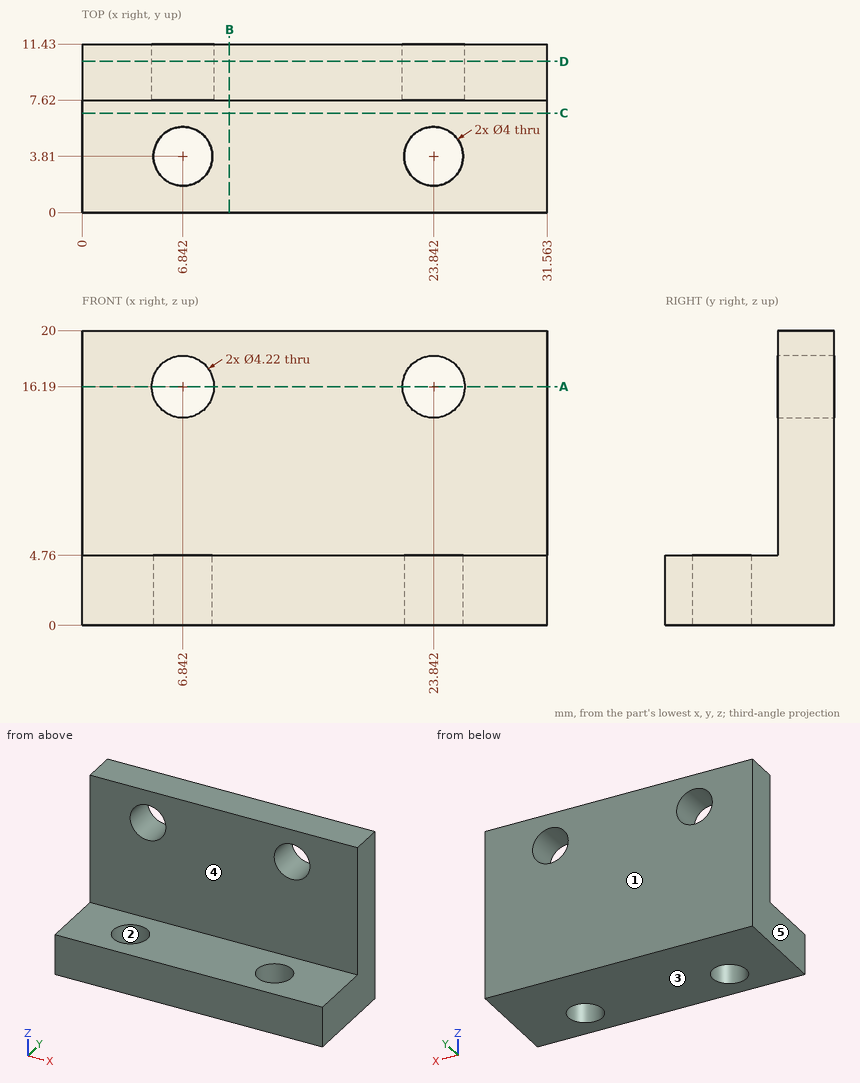
Input: dimensioned drawing with shaded views. Units: mm. Origin: part minimum x, y, z. A direction names the side the tool comes from. Round coordinates to 2 decimals unless told otherwise and drop trailing zeros. Write each loop counter-clockwise with the first axis right and the second up, starting at its lowest first coordinate (ties: lowest second). Pieces come first, ordered by that corner, then holes. Notation, with made-up numbers: (86.5, -12.5) - (136.5, -12.5) arc R18 cw to (136.5, -3.5) - close; hole circle Ø4 at (67.5, -38.5). An arc over 180 degrees is marked (long way). Write item = value, one per line.
(1) Pull-direction query (Y, two-part tool) for the marked faces 1, 2 and 3; classes: +Y half, -Y half, draft (parallel to the pull), parting line (faces both ways), or undercut.
Geometry check:
face_1 = +Y half
face_2 = undercut
face_3 = draft
(2) Contact query for a flat-ended pin moving along its axis: pin 1 Ø12 at (x, z) = (13, 11) entering from -Y. Output: stop coordinate, or through.
Geometry check:
pin_1 = 7.62
(3) Access query for the marked faces 4 and 5. Directions: +Z, -Z, +X, -X, +Y, -Y. A direction counts if a zero-diameter tool reaches every point of the face in a straight line with its end or side. Return the directions, or none.
Geometry check:
face_4 = +Z, +X, -X, -Y
face_5 = +Z, -Z, -X, +Y, -Y
(4) Section query D-D on y = 10.25. Output: boundary loops of the cut face in (x, z), then the cut area to 3 significant figures.
Geometry check:
outline = (0, 0) - (31.56, 0) - (31.56, 20) - (0, 20) - close; hole circle Ø4.22 at (6.84, 16.19); hole circle Ø4.22 at (23.84, 16.19)
area = 603 mm^2
(5) Section query C-C on y = 6.75. Output: boundary loops of the cut face in (x, z), then the cut area to 3 significant figures.
Geometry check:
outline = (0, 0) - (31.56, 0) - (31.56, 4.76) - (0, 4.76) - close
area = 150 mm^2
(6) Material intervals for probe 1 along X at (y, z) = (9.3, 16.19); probe 2 along X at (y, z) = (3.75, 1.25); probe 3 along Z at (x, y) = (6, 1.25), sorted ascending.
Geometry check:
probe_1 = 0 to 4.73, 8.95 to 21.73, 25.95 to 31.56
probe_2 = 0 to 4.84, 8.84 to 21.84, 25.84 to 31.56
probe_3 = 0 to 4.76
(7) Section query B-B on x = 10. Output: boundary loops of the cut face in (y, z).
Geometry check:
outline = (0, 0) - (11.43, 0) - (11.43, 20) - (7.62, 20) - (7.62, 4.76) - (0, 4.76) - close
(8) Section query A-A on z = 16.19. Output: boundary loops of the cut face in (x, y).
Geometry check:
outline = (0, 7.62) - (4.73, 7.62) - (4.73, 11.43) - (0, 11.43) - close; (8.95, 7.62) - (21.73, 7.62) - (21.73, 11.43) - (8.95, 11.43) - close; (25.95, 7.62) - (31.56, 7.62) - (31.56, 11.43) - (25.95, 11.43) - close
